```python
from build123d import *

# Parameters (mm, degrees)
SKETCH1_R      = 4.7752
SKETCH1_R_2    = 3.429
EXTRUDE1_DEPTH = 3.175
CHAMFER1_SIZE  = 0.254


with BuildPart() as part:
    # Sketch1 → Extrude1 (new body, symmetric)
    with BuildSketch(Plane.XY):
        Circle(SKETCH1_R)
        Circle(SKETCH1_R_2, mode=Mode.SUBTRACT)
    extrude(amount=EXTRUDE1_DEPTH, both=True)

    # Chamfer1
    chamfer1_edges = [part.edges().sort_by_distance(p)[0] for p in [
        (-4.7752, 0, -3.175),
        (-4.7752, 0, 3.175),
        (-3.429, 0, -3.175),
        (-3.429, 0, 3.175),
    ]]
    chamfer(chamfer1_edges, length=CHAMFER1_SIZE)


solid = part.part
```
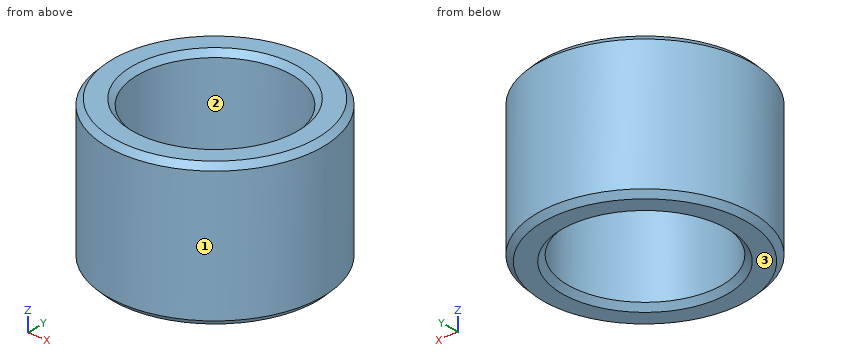
The model under review builds one solid part; all positions refer to its coordinate system, in mm. Face numbers are marked on the shaded views. Coordinates: 2 decimals unless noted, no trailing zeros. Order: outer loops, then holes, each group sorted by start corner. A loop starts at its lowest first (then second) coordinate and runs counter-clockwise, first axis right, second up. Notation, with made-up numbers: M 26.25,-27 L 40.25,-27 A30 ccw 40.25,0 Z; hole C -29.75,56 d10. An arc over 180 degrees is marked long. One line per question, with ' | ' between items.
(1) Insertion check: pin 1 (1.5 mm diameter, centred on x = -1.5, z = -1.5, fed in from -Y). The pin has a flat end and moves straight along its axis. Give the tip position at first contact, or say it passes through.
Geometry results:
pin 1: stops at y = -4.72
(2) Add section C-C, the plane z = 2.5. Write out the cut boundary in (x, y), then the cut area to 3 significant figures.
Geometry results:
outline: C 0,0 d9.55; hole C 0,0 d6.86 | area: 34.7 mm²
(3) For probe 1 along Y at (x, z) = (0, -1.35); probe 2 along Y at (x, z) = (-1, 1.5); probe 3 along X at (y, z) = (2, 0.75), list the stretches that pass through material, from the lowest coordinate up. Write a range as from..to.
Geometry results:
probe 1: y = -4.78..-3.43, 3.43..4.78 | probe 2: y = -4.67..-3.28, 3.28..4.67 | probe 3: x = -4.34..-2.79, 2.79..4.34
(4) The part is to be moulded in two halves that separate along Y. For the marked faces 1, 2 and 3, say which applies: +Y half, -Y half, draft (parallel to the pull), parting line (faces both ways), or undercut.
Geometry results:
face 1: parting line | face 2: undercut | face 3: draft
(5) Add section A-A, the plane x = 0. Write out the cut boundary in (y, z) (3 decimals), then the cut area to 3 significant figures.
Geometry results:
outline: M -4.775,-2.921 L -4.521,-3.175 L -3.683,-3.175 L -3.429,-2.921 L -3.429,2.921 L -3.683,3.175 L -4.521,3.175 L -4.775,2.921 Z; M 3.429,-2.921 L 3.683,-3.175 L 4.521,-3.175 L 4.775,-2.921 L 4.775,2.921 L 4.521,3.175 L 3.683,3.175 L 3.429,2.921 Z | area: 16.8 mm²
